Build history of the part. All positions in model axes, mm. A direction names the side the tool comes from. Give positions to 0.01 mm unless a question says otherwise; leave off trailing zeros. Order: outer loops, then holes, each group sorted by start corner. A loop starts at its lowest first (then second) coordinate and runs counter-clockwise, first axis right, second up. Notation, with made-up numbers: (21.5, 31) -> (47.5, 31) arc R14 cw to (47.5, 35) -> close; hole circle Ø7 at (-12.5, 70). An arc over 180 degrees is marked (long way). One line per item, written item: value. Start each with the question number.
(1) Saw through at B-B on x = 503. Give the cut face in (y, z).
(2) Saw through at A-A on z = -270. Give the cut face in (x, y), plus the area to 4 significant figures.
(3) Which spindle directions (+Z, -Z, +X, -X, +Y, -Y) get a long thin tool onto all of the face, cutting with end or side? Do faces 1 (the flat face through (175, 6, -177)), 2 (the flat face through (530, 5, -177)). Say none if no direction does.
(4) Pin check, flat tips, straight feed: pin 1 (1.1 mm diameter, centred on y = 5.5, z = -111.5, fed in from +X); pin 2 (1.5 mm diameter, centred on x = 592, z = -181.5, fed in from +Y). Stop position of each tip, or through.
(5) Probe line 1 (X direction, y = 5.5, z = -132); line 2 (Y direction, x = 596.5, z = -91.5); line 3 (X direction, y = 3.5, z = -332). List the from-to ranges inside material, lowest first.
```python
from build123d import *

# Parameters (mm, degrees)
SKETCH1_W           = 710
SKETCH1_H           = 350
BOSS_EXTRUDE1_DEPTH = 5
SKETCH2_W           = 355
SKETCH2_H           = 350
BOSS_EXTRUDE2_DEPTH = 1
CUT_EXTRUDE1_DEPTH  = 792.603436071


with BuildPart() as part:
    # Sketch1 → Boss-Extrude1 (new body)
    with BuildSketch(Plane(origin=(0, 0, 0), x_dir=(1, 0, 0), z_dir=(0, 1, 0))):
        with Locations((355, 175)):
            Rectangle(SKETCH1_W, SKETCH1_H)
    extrude(amount=BOSS_EXTRUDE1_DEPTH)

    # Sketch2 → Boss-Extrude2 (add)
    with BuildSketch(Plane(origin=(0, 5, 0), x_dir=(1, 0, 0), z_dir=(0, 1, 0))):
        with Locations((177.5, 175)):
            Rectangle(SKETCH2_W, SKETCH2_H)
    extrude(amount=BOSS_EXTRUDE2_DEPTH)

    # Sketch3 → Cut-Extrude1 (cut, through all)
    with BuildSketch(Plane(origin=(0, 6, 0), x_dir=(1, 0, 0), z_dir=(0, 1, 0))):
        Polygon((0, 350), (0, 315), (35, 350), align=None)
        Polygon((35, 0), (0, 35), (0, 0), align=None)
    extrude(amount=-CUT_EXTRUDE1_DEPTH, mode=Mode.SUBTRACT)


solid = part.part
```
Results below:
1. outline: (0, -350) -> (5, -350) -> (5, 0) -> (0, 0) -> close
2. outline: (0, 0) -> (710, 0) -> (710, 5) -> (355, 5) -> (355, 6) -> (0, 6) -> close
2. area: 3,905 mm²
3. face 1: +Z, -Z, +X, -X, +Y
3. face 2: +Z, -Z, +X, +Y
4. pin 1: stops at x = 710
4. pin 2: stops at y = 5
5. line 1: x = 0 to 355
5. line 2: y = 0 to 5
5. line 3: x = 17 to 710
